from build123d import *

# Parameters (mm, degrees)
F0_R     = 7.5
F0_R_2   = 4
F1_DEPTH = 3.25
F2_R     = 7
F2_R_2   = 4
F3_DEPTH = 1
F4_R     = 7.5
F4_R_2   = 7
F4_R_3   = 4
F5_DEPTH = 15.5
F6_R     = 7
F6_R_2   = 4
F7_DEPTH = 1
F8_R     = 7.5
F8_R_2   = 7
F8_R_3   = 4
F9_DEPTH = 3.25


# Not quite as in the source:
# - a feature names something its author has since deleted; it is built from what else it names


with BuildPart() as f1:
    # F0 (on Front) → F1 (new body)
    with BuildSketch(Plane.XZ):
        Circle(F0_R)
        Circle(F0_R_2, mode=Mode.SUBTRACT)
    extrude(amount=F1_DEPTH)

    # F2 (on face) → F3 (join)
    with BuildSketch(Plane.XZ.offset(3.25)):
        Circle(F2_R)
        Circle(F2_R_2, mode=Mode.SUBTRACT)
    extrude(amount=F3_DEPTH)

    # F4 (on face) → F5 (join)
    with BuildSketch(Plane.XZ.offset(4.25)):
        Circle(F4_R)
        Circle(F4_R_2, mode=Mode.SUBTRACT)
        Circle(F4_R_2)
        Circle(F4_R_3, mode=Mode.SUBTRACT)
    extrude(amount=F5_DEPTH)

    # F6 (on face) → F7 (join)
    with BuildSketch(Plane.XZ.offset(19.75)):
        Circle(F6_R)
        Circle(F6_R_2, mode=Mode.SUBTRACT)
    extrude(amount=F7_DEPTH)

    # F8 (on face) → F9 (join)
    with BuildSketch(Plane.XZ.offset(20.75)):
        Circle(F8_R)
        Circle(F8_R_2, mode=Mode.SUBTRACT)
        Circle(F8_R_2)
        Circle(F8_R_3, mode=Mode.SUBTRACT)
    extrude(amount=F9_DEPTH)


solid = f1.part
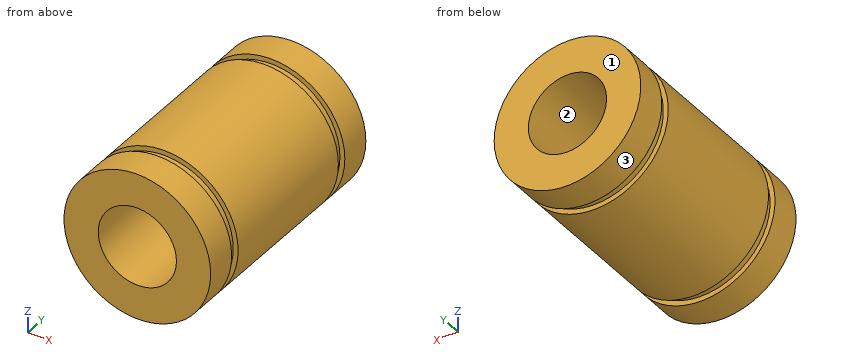
Input: part model. Units: mm. Frame: model coordinates. Face numbers are marked on the shaded views. Coordinates: 2 decimals unless noted, no trailing zeros. Loops run counter-clockwise (first coordinate to the right, second up) from the corner with the lowest first, then second, coordinate; pieces in that order, holes last. Notation, with made-up numbers: (9, 62.25) -> (35, 62.25) arc R12 ccw to (35, 72.25) -> close; hole circle Ø2 at (36, 44.25). An arc over 180 degrees is marked (long way). Write each question's results on one line, items separated by ' | '. Start each with the question number.
Q1. Pin query (flat end, axial travel): pin 1 (1.5 mm diameter, centred on x = 2, y = -17.5, fed in from -Z); pin 2 (1 mm diameter, centred on x = 0.5, z = -1.5, fed in from +Y); pin 3 (5 mm diameter, centred on x = -4, y = -17.5, fed in from -Z). Return the tip coordinate at first contact, or that it passes through.
Q2. Section A-A, the plane z = -3. Return the cut outline in (x, y), plus the area to 3 significant figures.
Q3. Section C-C, the plane x = -5.5. Return the cut outline in (y, z), plus the area to 3 significant figures.
Q4. Section B-B, the plane x = 0. Return the cut outline in (y, z).
Q5. Pull-direction query (Z, two-part tool) for the marked faces 1, 2 and 3; classes: released by +Z, released by -Z, zero draft, split by the parting line, or undercut.
Q6. Section D-D, the plane y = -11.25. Return the cut outline in (x, z), plus the area to 3 significant figures.
Q7. Ray query, line 1 (Y direction, x = 4, z = 6.25); line 2 (Z direction, x = 0, y = -16.75); line 3 (Z direction, x = 2.75, y = -16.25). Return the intervals inside material, ascending. Write a range as from..to.
Found:
1) pin 1: z = -7.4 | pin 2: through | pin 3: z = -7.35
2) outline: (-6.87, -24) -> (-2.65, -24) -> (-2.65, 0) -> (-6.87, 0) -> (-6.87, -3.25) -> (-6.32, -3.25) -> (-6.32, -4.25) -> (-6.87, -4.25) -> (-6.87, -19.75) -> (-6.32, -19.75) -> (-6.32, -20.75) -> (-6.87, -20.75) -> close; (2.65, -24) -> (6.87, -24) -> (6.87, -20.75) -> (6.32, -20.75) -> (6.32, -19.75) -> (6.87, -19.75) -> (6.87, -4.25) -> (6.32, -4.25) -> (6.32, -3.25) -> (6.87, -3.25) -> (6.87, 0) -> (2.65, 0) -> close | area: 201 mm2
3) outline: (-24, -5.1) -> (-20.75, -5.1) -> (-20.75, -4.33) -> (-19.75, -4.33) -> (-19.75, -5.1) -> (-4.25, -5.1) -> (-4.25, -4.33) -> (-3.25, -4.33) -> (-3.25, -5.1) -> (0, -5.1) -> (0, 5.1) -> (-3.25, 5.1) -> (-3.25, 4.33) -> (-4.25, 4.33) -> (-4.25, 5.1) -> (-19.75, 5.1) -> (-19.75, 4.33) -> (-20.75, 4.33) -> (-20.75, 5.1) -> (-24, 5.1) -> close | area: 242 mm2
4) outline: (-24, -7.5) -> (-20.75, -7.5) -> (-20.75, -7) -> (-19.75, -7) -> (-19.75, -7.5) -> (-4.25, -7.5) -> (-4.25, -7) -> (-3.25, -7) -> (-3.25, -7.5) -> (0, -7.5) -> (0, -4) -> (-24, -4) -> close; (-24, 4) -> (0, 4) -> (0, 7.5) -> (-3.25, 7.5) -> (-3.25, 7) -> (-4.25, 7) -> (-4.25, 7.5) -> (-19.75, 7.5) -> (-19.75, 7) -> (-20.75, 7) -> (-20.75, 7.5) -> (-24, 7.5) -> close
5) face 1: zero draft | face 2: undercut | face 3: split by the parting line
6) outline: circle Ø15 at (0, 0); hole circle Ø8 at (0, 0) | area: 126 mm2
7) line 1: -24..-20.75, -19.75..-4.25, -3.25..0 | line 2: -7.5..-4, 4..7.5 | line 3: -6.98..-2.9, 2.9..6.98
